from build123d import *

# Parameters (mm, degrees)
SKETCH1_W           = 100
SKETCH1_H           = 100
SKETCH1_R           = 3.25
BOSS_EXTRUDE1_DEPTH = 16
SKETCH2_R           = 8
CUT_EXTRUDE1_DEPTH  = 8
CUT_EXTRUDE2_REACH  = 10
SKETCH3_R           = 6.4


with BuildPart() as part:
    # Sketch1 → Boss-Extrude1 (new body)
    with BuildSketch(Plane(origin=(0, 0, 0), x_dir=(1, 0, 0), z_dir=(0, 1, 0))):
        Rectangle(SKETCH1_W, SKETCH1_H)
        Circle(SKETCH1_R, mode=Mode.SUBTRACT)
    extrude(amount=BOSS_EXTRUDE1_DEPTH)

    # Sketch2 → Cut-Extrude1 (cut)
    with BuildSketch(Plane(origin=(0, 16, 0), x_dir=(1, 0, 0), z_dir=(0, 1, 0))):
        with Locations((0, -25)):
            Circle(SKETCH2_R)
    extrude(amount=-CUT_EXTRUDE1_DEPTH, mode=Mode.SUBTRACT)

    # Sketch3 → Cut-Extrude2 (cut, up to next)
    with BuildSketch(Plane(origin=(0, 8, 0), x_dir=(1, 0, 0), z_dir=(0, 1, 0)), mode=Mode.PRIVATE) as cut_extrude2_sk1:
        with Locations((0, -25)):
            Circle(SKETCH3_R)
    cut_extrude2_tool1 = extrude(cut_extrude2_sk1.sketch, amount=-CUT_EXTRUDE2_REACH, mode=Mode.PRIVATE) & part.part
    add(cut_extrude2_tool1.solids().sort_by_distance((0, 8, 25))[0], mode=Mode.SUBTRACT)


solid = part.part
Check sheet for the modelled part. Datum: model origin and axes. Units: mm. A direction names the side the tool comes from. Round coordinates to 2 decimals unless told otherwise and drop trailing zeros. Loops run counter-clockwise (first coordinate to the right, second up) from the corner with the lowest first, then second, coordinate; pieces in that order, holes last. Notation, with made-up numbers: M 79.5,46.25 L 113.5,46.25 A23 ccw 113.5,68.25 Z; hole C -35,46 d1. An arc over 180 degrees is marked long. One line per item, written item: value.
(1) Sectioned sample at D-D, the plane z = 25. Record the cut outline in (x, y).
Computed values:
outline: M -50,0 L -6.4,0 L -6.4,8 L -8,8 L -8,16 L -50,16 Z; M 6.4,0 L 50,0 L 50,16 L 8,16 L 8,8 L 6.4,8 Z
(2) Release check for a two-part mould opening along Z. For faces 3 (the face through (-1, 8, -50)), 4 (the face through (-1.73, 12.06, 32.81)), 5 (the face through (-50, 8, 1)) record: +Z half, -Z half, draft (parallel to the pull), parting line (faces both ways), or undercut.
Computed values:
face 3: -Z half
face 4: undercut
face 5: draft
(3) Sectioned sample at B-B, the plane z = 0. Record the cut outline in (x, y).
Computed values:
outline: M -50,0 L -3.25,0 L -3.25,16 L -50,16 Z; M 3.25,0 L 50,0 L 50,16 L 3.25,16 Z
(4) Thickness scan on line 1 (Z direction, x = 0, y = 6.25); line 2 (Z direction, x = 0, y = 11.5); line 3 (X direction, y = 10.5, z = 25). Record the ranges inside material, lowest first.
Computed values:
line 1: z = -50 to -3.25, 3.25 to 18.6, 31.4 to 50
line 2: z = -50 to -3.25, 3.25 to 17, 33 to 50
line 3: x = -50 to -8, 8 to 50
(5) Access from +Z, -Z, +X, -X, +Y, -Y to the whole of each face (thin tool, end or side, straight path). Record for faces 1 (the face through (-1, 16, -12)), 2 (the face through (0, 8, 18)).
Computed values:
face 1: +Z, -Z, +X, -X, +Y
face 2: +Y
(6) Sectioned sample at A-A, the plane x = 0. Record the cut outline in (y, z), then the cut area to 3 significant figures.
Computed values:
outline: M 0,-50 L 16,-50 L 16,-3.25 L 0,-3.25 Z; M 0,3.25 L 16,3.25 L 16,17 L 8,17 L 8,18.6 L 0,18.6 Z; M 0,31.4 L 8,31.4 L 8,33 L 16,33 L 16,50 L 0,50 Z
area: 1,270 mm^2
(7) Depth check by flat-ended pin: pin 1 Ø10 at (x, z) = (0, 25) entering from -Y; pin 2 Ø14.5 at (x, z) = (0, 25) entering from +Y; pin 3 Ø1 at (x, z) = (9.5, 23.5) entering from -Y. Enter the tip coordinate at first touch or a pass-through.
Computed values:
pin 1: passes through
pin 2: stops at y = 8
pin 3: stops at y = 0
(8) Sectioned sample at C-C, the plane y = 12.75. Record the cut outline in (x, z), then the cut area to 3 significant figures.
Computed values:
outline: M -50,-50 L 50,-50 L 50,50 L -50,50 Z; hole C 0,25 d16; hole C 0,0 d6.5
area: 9,770 mm^2
